Design review of the part built by this model. Coordinates are the model's own, in mm. A direction names the side the tool comes from. Round coordinates to 2 decimals unless told otherwise and drop trailing zeros. Order: outer loops, then holes, each group sorted by start corner. A loop starts at its lowest first (then second) coordinate and runs counter-clockwise, first axis right, second up. Notation, with made-up numbers: (46.25, -39) - (80.25, -39) arc R13 ccw to (80.25, -22) - close; hole circle Ø7 at (67.5, -4). An arc over 180 degrees is marked (long way). Use CSV: the item, a comma, the result in double quotes.
from build123d import *

# Parameters (mm, degrees)
BOSS_EXTRUDE2_DEPTH     = 13.9
CUT_EXTRUDE1_DEPTH      = 21.451161336
CUT_EXTRUDE1_DEPTH_BACK = 21.451161336
SKETCH2_R               = 1.15
SKETCH3_R               = 1.45
CUT_EXTRUDE2_DEPTH      = 28.025358462
FILLET1_R               = 3.8


with BuildPart() as part:
    # Sketch1 → Boss-Extrude2 (new body)
    with BuildSketch(Plane.XY):
        Polygon((-8, 10.2), (-8, 5), (8, 5), (8, -5), (-8, -5), (-8, -10.2), (11, -10.2), (11, 10.2), align=None)
    extrude(amount=-BOSS_EXTRUDE2_DEPTH)

    # Sketch2 → Cut-Extrude1 (cut, two sides: drawn at the far end of the back side and taken through both)
    with BuildSketch(Plane.XY.offset(-CUT_EXTRUDE1_DEPTH_BACK)):
        with Locations((5, 7.6)):
            Circle(SKETCH2_R)
        with Locations((5, -7.6)):
            Circle(SKETCH2_R)
    extrude(amount=CUT_EXTRUDE1_DEPTH + CUT_EXTRUDE1_DEPTH_BACK, mode=Mode.SUBTRACT)

    # Sketch3 → Cut-Extrude2 (cut, through all)
    with BuildSketch(Plane(origin=(0, 10.2, 0), x_dir=(1, 0, 0), z_dir=(0, 1, 0))):
        with Locations(Location((0, 6.95, 0), (0, 0, 180))):
            Circle(SKETCH3_R)
    extrude(amount=-CUT_EXTRUDE2_DEPTH, mode=Mode.SUBTRACT)

    # Fillet1
    fillet1_edges = [part.edges().sort_by_distance(p)[0] for p in [
        (-8, -10.2, -6.95),
        (-8, 10.2, -6.95),
    ]]
    fillet(fillet1_edges, radius=FILLET1_R)


solid = part.part
1) We need section B-B (x = -2.5). Give the boundary of the cut face in (y, z), then the cut area to 3 significant figures.
Data:
outline,"(-10.2, -13.9) - (-5, -13.9) - (-5, 0) - (-10.2, 0) - close; (5, -13.9) - (10.2, -13.9) - (10.2, 0) - (5, 0) - close"
area,"145 mm2"
2) We need section A-A (z = -6.95). Give the boundary of the cut face in (x, y), then the cut area to 3 significant figures.
Data:
outline,"(-8, -6.4) arc R3.8 ccw to (-4.2, -10.2) - (-1.45, -10.2) - (-1.45, -5) - (-8, -5) - close; (-8, 5) - (-1.45, 5) - (-1.45, 10.2) - (-4.2, 10.2) arc R3.8 ccw to (-8, 6.4) - close; (1.45, -10.2) - (11, -10.2) - (11, 10.2) - (1.45, 10.2) - (1.45, 5) - (8, 5) - (8, -5) - (1.45, -5) - close; hole circle Ø2.3 at (5, -7.6); hole circle Ø2.3 at (5, 7.6)"
area,"183 mm2"
3) For faces 1 (the face through (11, 0, -7)), 2 (the face through (0, -5, -5)), list the 3-axis set-ups (+Z, -Z, +X, -X, +Y, -Y) from which the entire face can be reached by the end or side of a thin tool; tool diameter is ignored.
Data:
face 1,"+Z, -Z, +X, +Y, -Y"
face 2,"+Z, -Z, -X"
4) To check wall thickness, follow L1, parallel to Y at x = 5, z = -4; L2, parallel to Y at x = -3.25, z = -4.5; L3, parallel to X at y = 7.6, z = -7. State the ranges of each line that lie inside material, in increasing order. Write a range as from..to.
Data:
L1,"y = -10.2..-8.75, -6.45..-5, 5..6.45, 8.75..10.2"
L2,"y = -10.2..-5, 5..10.2"
L3,"x = -7.81..-1.45, 1.45..3.85, 6.15..11"
5) Insertion check: pin 1 Ø3 at (x, y) = (5, 7.6) entering from -Z; pin 2 Ø3 at (y, z) = (-3, -3.5) entering from -X. Each pin has a flat end and moves straight along its axis. Give the tip position at first contact, or say it passes through.
Data:
pin 1,"stops at z = -13.9"
pin 2,"stops at x = 8"
6) The part is to be moulded in two halves that separate along Z. For faces 3 (the face through (0, 5, -5)), 4 (the face through (3, 7, 0)), 5 (the face through (0.189, 7.636, -5.512)), say which applies: +Z half, -Z half, draft (parallel to the pull), parting line (faces both ways), or undercut.
Data:
face 3,"draft"
face 4,"+Z half"
face 5,"undercut"
7) We need section C-C (y = 7). Give the boundary of the cut face in (x, z).
Data:
outline,"(-7.95, -13.9) - (4.02, -13.9) - (4.02, 0) - (-7.95, 0) - close; (5.98, -13.9) - (11, -13.9) - (11, 0) - (5.98, 0) - close; hole circle Ø2.9 at (0, -6.95)"
8) We need section D-D (z = -12.25). Give the boundary of the cut face in (x, y), then the cut area to 3 significant figures.
Data:
outline,"(-8, -6.4) arc R3.8 ccw to (-4.2, -10.2) - (11, -10.2) - (11, 10.2) - (-4.2, 10.2) arc R3.8 ccw to (-8, 6.4) - (-8, 5) - (8, 5) - (8, -5) - (-8, -5) - close; hole circle Ø2.3 at (5, -7.6); hole circle Ø2.3 at (5, 7.6)"
area,"213 mm2"
